CAD build for the part. Positions are in the model's coordinates, mm. Face numbers are marked on the shaded views. A direction names the side the tool comes from. Coordinates: 2 decimals unless noted, no trailing zeros. Order: outer loops, then holes, each group sorted by start corner. A loop starts at its lowest first (then second) coordinate and runs counter-clockwise, first axis right, second up. Notation, with made-up numbers: (11, -4) - (69, -4) arc R13 ccw to (69, 0) - close; hole circle Ø4 at (-12, 43.5). An arc over 180 degrees is marked (long way). Use one line per item in the form item = value.
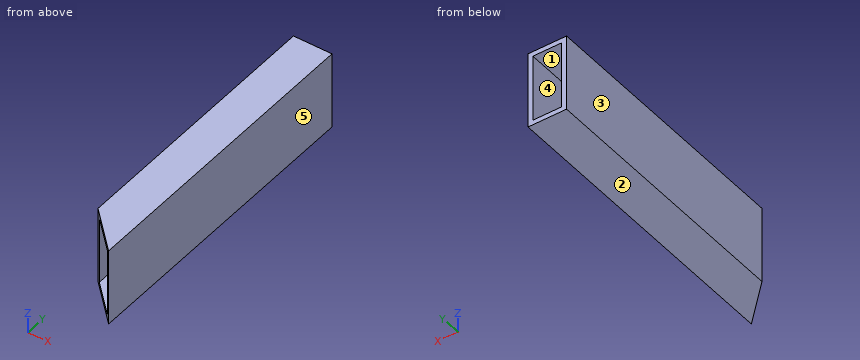
```python
from build123d import *

# Parameters (mm, degrees)
F0_W        = 25.4
F0_H        = 50.8
F0_W_2      = 19.05
F0_H_2      = 44.45
F1_DEPTH    = 203.2
F2_T1_DEPTH = 181.4414957887


# Not quite as in the source:
# - a fillet or chamfer that OpenCascade refuses, or shapes differently, is made with other operations: its cross-section is extruded or revolved along the edge and cut away or added


with BuildPart() as f1:
    # F0 (on Front) → F1 (new body)
    with BuildSketch(Plane.XZ):
        with Locations((0, 11.1125)):
            Rectangle(F0_W, F0_H)
        with Locations((0, 11.1125)):
            Rectangle(F0_W_2, F0_H_2, mode=Mode.SUBTRACT)
    extrude(amount=F1_DEPTH)

    # F2: chamfer of 25.4 on 1 edges, made by hand

    # F2_s2 → F2_t1 (cut)
    with BuildSketch(Plane.XY.offset(-79.6082478943)):
        Polygon((-12.7, -177.8), (12.7, -203.2), (-12.7, -203.2), align=None)
    extrude(amount=F2_T1_DEPTH, mode=Mode.SUBTRACT)


solid = f1.part
```
Item 1: Two-plate mould, pull along Z, no slides. Class the marked faces 1, 2 and 3: +Z half, -Z half, draft (parallel to the pull), parting line (faces both ways), or undercut.
Derived:
face_1 = undercut
face_2 = -Z half
face_3 = draft
Item 2: 3-axis set-ups, long thin cutter, end or side, ignore diameter. For the marked faces 4 and 5: which of +Z, -Z, +X, -X, +Y, -Y reach the whole face in a straight line?
Derived:
face_4 = +Y, -Y
face_5 = +Z, -Z, +X, +Y, -Y
Item 3: Cut at C-C, the plane y = -92.5. Write the cut outline in (x, z) (1 decimal).
Derived:
outline = (-12.7, -14.3) - (12.7, -14.3) - (12.7, 36.5) - (-12.7, 36.5) - close; hole (-9.5, -11.1) - (9.5, -11.1) - (9.5, 33.3) - (-9.5, 33.3) - close
Item 4: Cut at B-B, the plane z = 22. Write the cut outline in (x, y) (3 decimals).
Derived:
outline = (-12.7, -177.8) - (-9.525, -180.975) - (-9.525, 0) - (-12.7, 0) - close; (9.525, -200.025) - (12.7, -203.2) - (12.7, 0) - (9.525, 0) - close
Item 5: Drill centre lines: line 1 (X direction, y = -102.5, z = 8) (3 decimals); line 2 (Z direction, x = 2, y = -119.5); line 3 (Y direction, x = 1.5, z = 33.5). Where is each one in solid material? Low to high. Write a range as [from, to].
Derived:
line_1 = [-12.7, -9.525], [9.525, 12.7]
line_2 = [-14.29, -11.11], [33.34, 36.51]
line_3 = [-192, 0]
Item 6: Cut at A-A, the plane x = 5.75. Write the cut outline in (y, z).
Derived:
outline = (-196.25, -14.29) - (0, -14.29) - (0, -11.11) - (-196.25, -11.11) - close; (-196.25, 33.34) - (0, 33.34) - (0, 36.51) - (-196.25, 36.51) - close
